```python
from build123d import *

# Parameters (mm, degrees)
ESBO_O1_W       = 16
ESBO_O1_H       = 52
ESBO_O1_R       = 4
EXTRUS_O1_DEPTH = 2.5


with BuildPart() as part:
    # Esboço1 → Extrusão1 (new, symmetric)
    with BuildSketch(Plane.XY):
        with Locations((0, 4)):
            Rectangle(ESBO_O1_W, ESBO_O1_H)
        Circle(ESBO_O1_R, mode=Mode.SUBTRACT)
    extrude(amount=EXTRUS_O1_DEPTH, both=True)


solid = part.part
```
Input: part model. Units: mm. Frame: model coordinates. Round coordinates to 2 decimals unless told otherwise and drop trailing zeros. Loops run counter-clockwise (first coordinate to the right, second up) from the corner with the lowest first, then second, coordinate; pieces in that order, holes last. Notation, with made-up numbers: (56.25, 75) -> (103.25, 75) arc R30 cw to (103.25, 105) -> close; hole circle Ø4 at (54.5, 69). An arc over 180 degrees is marked (long way). Use one line per item in the form item = value. Start each with the question number.
Item 1: Mould query, pull axis Y, two halves, no side actions, for faces 1 (the face through (-0.1, 4.4, 2.5)), 2 (the face through (0, -22, 0)), 3 (the face through (-0.867, -3.905, -0.035)), 4 (the face through (0, 30, 0)). Classes: pulls with the +Y half, pulls with the -Y half, needs draft (parallel to the pull), parting line crosses it, or undercut.
Item 2: Section query A-A on x = 0. Return the cut outline in (y, z), then the cut area to 3 significant figures.
Item 3: Section query B-B on z = -1.8. Return the cut outline in (x, y).
Item 4: Material intervals for L1, parallel to Y at x = 0, z = -1; L2, parallel to Y at x = -1.75, z = 0.4; L3, parallel to X at y = 3.5, z = 1.65, sorted ascending. Write a range as from..to.
Item 5: Section query C-C on x = 2. Return the cut outline in (y, z), then the cut area to 3 significant figures.
Ans:
q1.face_1 = needs draft
q1.face_2 = pulls with the -Y half
q1.face_3 = undercut
q1.face_4 = pulls with the +Y half
q2.outline = (-22, -2.5) -> (-4, -2.5) -> (-4, 2.5) -> (-22, 2.5) -> close; (4, -2.5) -> (30, -2.5) -> (30, 2.5) -> (4, 2.5) -> close
q2.area = 220 mm^2
q3.outline = (-8, -22) -> (8, -22) -> (8, 30) -> (-8, 30) -> close; hole circle Ø8 at (0, 0)
q4.L1 = -22..-4, 4..30
q4.L2 = -22..-3.6, 3.6..30
q4.L3 = -8..-1.94, 1.94..8
q5.outline = (-22, -2.5) -> (-3.46, -2.5) -> (-3.46, 2.5) -> (-22, 2.5) -> close; (3.46, -2.5) -> (30, -2.5) -> (30, 2.5) -> (3.46, 2.5) -> close
q5.area = 225 mm^2
